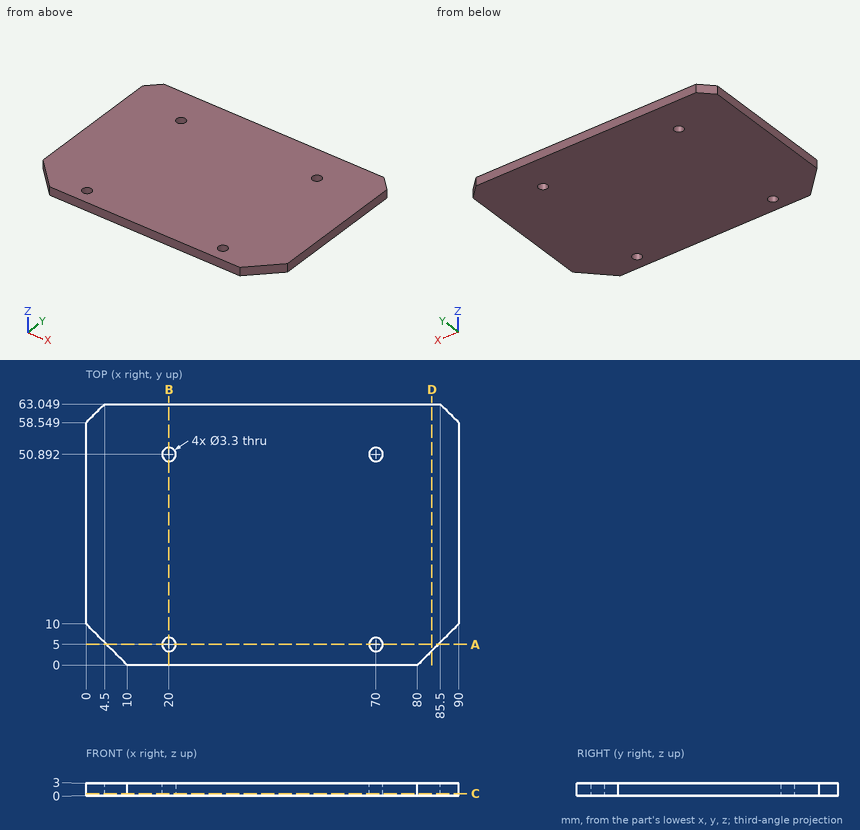
Source: three-view drawing plus pictorial views. Frame: mm from the lowest corner of the part. Coordinates: 2 decimals unless noted, no trailing zeros. Write each loop counter-clockwise with the first axis right and the second up, starting at its lowest first coordinate (ties: lowest second). Pieces come first, ordered by that corner, then holes. Notation, with made-up numbers: (0.5, -6.5) - (47.5, -6.5) arc R22 cw to (47.5, 28.5) - close; hole circle Ø11 at (31.25, -26.75). An arc over 180 degrees is marked (long way). Answer as a JSON object with one key per item and string values.
Q1. Section query A-A, the plane y = 5. Output: boundary loops of the cut face in (x, z), plus the area to 3 significant figures.
Ans:
{"outline": "(5, 0) - (18.35, 0) - (18.35, 3) - (5, 3) - close; (21.65, 0) - (68.35, 0) - (68.35, 3) - (21.65, 3) - close; (71.65, 0) - (85, 0) - (85, 3) - (71.65, 3) - close", "area": "220 mm2"}
Q2. Section query C-C, the plane z = 0.5. Output: boundary loops of the cut face in (x, y), plus the area to 3 significant figures.
Ans:
{"outline": "(0, 10) - (10, 0) - (80, 0) - (90, 10) - (90, 58.55) - (85.5, 63.05) - (4.5, 63.05) - (0, 58.55) - close; hole circle Ø3.3 at (20, 5); hole circle Ø3.3 at (20, 50.89); hole circle Ø3.3 at (70, 5); hole circle Ø3.3 at (70, 50.89)", "area": "5,520 mm2"}
Q3. Section query D-D, the plane x = 83.5. Output: boundary loops of the cut face in (y, z), plus the area to 3 significant figures.
Ans:
{"outline": "(3.5, 0) - (63.05, 0) - (63.05, 3) - (3.5, 3) - close", "area": "179 mm2"}
Q4. Section query B-B, the plane x = 20. Output: boundary loops of the cut face in (y, z).
Ans:
{"outline": "(0, 0) - (3.35, 0) - (3.35, 3) - (0, 3) - close; (6.65, 0) - (49.24, 0) - (49.24, 3) - (6.65, 3) - close; (52.54, 0) - (63.05, 0) - (63.05, 3) - (52.54, 3) - close"}
Q5. First-contact query: pin 1 Ø1 at (x, z) = (49.5, 0.5) entering from -Y. Flat tip, straight axial feed; report the tip coordinate or a pass-through.
Ans:
{"pin 1": "stops at y = 0"}
Q6. Material intervals for line 1 (Y direction, x = 70, z = 1.6); line 2 (X direction, y = 4, z = 1.85), sorted ascending. Write a range as [from, to].
Ans:
{"line 1": "y = [0, 3.35], [6.65, 49.24], [52.54, 63.05]", "line 2": "x = [6, 18.69], [21.31, 68.69], [71.31, 84]"}
